from build123d import *

# Parameters (mm, degrees)
SKETCH1_R           = 25
SKETCH1_R_2         = 1.5
BOSS_EXTRUDE1_DEPTH = 7
FILLET1_R           = 0.4
BOSS_EXTRUDE2_DEPTH = 7
MOVE_FACE1_DEPTH    = 7


# Read off the part's stored shape, not the designer's step: Move Face1
with BuildPart() as part:
    # Sketch1 → Boss-Extrude1 (new body)
    with BuildSketch(Plane.XY):
        Circle(SKETCH1_R)
        Circle(SKETCH1_R_2, mode=Mode.SUBTRACT)
    extrude(amount=BOSS_EXTRUDE1_DEPTH)

    # Sketch2 → Cut-Revolve1 (revolve, cut)
    with BuildSketch(Plane(origin=(0, 0, 0), x_dir=(0, 0, -1), z_dir=(1, 0, 0)), mode=Mode.PRIVATE) as cut_revolve1_sk:
        with BuildLine():
            Line((-7, 25), (-6.139887117, 24.237039248))
            ThreePointArc((-6.139887117, 24.237039248), (-3.5, 23.102184954), (-0.860112883, 24.237039248))
            Line((-0.860112883, 24.237039248), (0, 25))
            Line((0, 25), (-7, 25))
        make_face()
    revolve(cut_revolve1_sk.sketch.rotate(Axis((0, 0, 7), (0, 0, -1)), 90), axis=Axis((0, 0, 7), (0, 0, -1)), mode=Mode.SUBTRACT)

    # Fillet1
    fillet1_edges = [part.edges().sort_by_distance(p)[0] for p in [
        (-25, 0, 0),
        (-25, 0, 7),
    ]]
    fillet(fillet1_edges, radius=FILLET1_R)

    # Sketch3 → Boss-Extrude2 (add, through all)
    with BuildSketch(Plane.XY.offset(7)):
        with BuildLine():
            Line((-1.12, 0.997797575), (1.12, 0.997797575))
            ThreePointArc((1.12, 0.997797575), (0, 1.5), (-1.12, 0.997797575))
        make_face()
    extrude(amount=-BOSS_EXTRUDE2_DEPTH)

    # Move Face1 outline → Move Face1 (cut)
    with BuildSketch(Plane.XY):
        with BuildLine():
            ThreePointArc((-1.314115672, 0.997797575), (0, -1.65), (1.314115672, 0.997797575))
            Line((1.314115672, 0.997797575), (1.12, 0.997797575))
            ThreePointArc((1.12, 0.997797575), (0, -1.5), (-1.12, 0.997797575))
            Line((-1.12, 0.997797575), (-1.314115672, 0.997797575))
        make_face()
    extrude(amount=MOVE_FACE1_DEPTH, mode=Mode.SUBTRACT)


solid = part.part
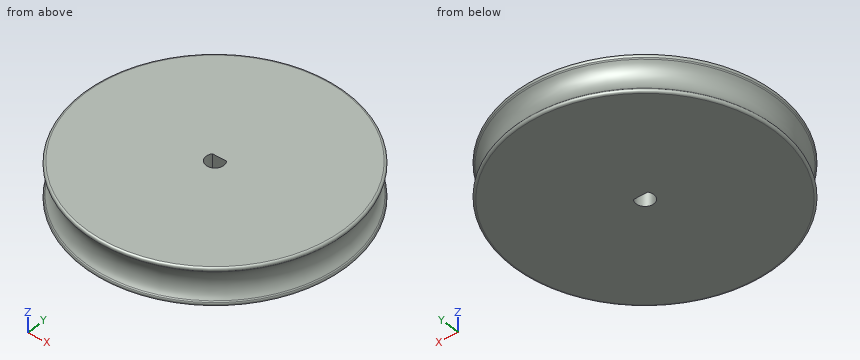
CAD build for the part. Positions are in the model's coordinates, mm. Round coordinates to 2 decimals unless told otherwise and drop trailing zeros. Order: outer loops, then holes, each group sorted by start corner. A loop starts at its lowest first (then second) coordinate and runs counter-clockwise, first axis right, second up. Notation, with made-up numbers: (22, 88.25) -> (41, 88.25) arc R18 cw to (41, 106.25) -> close; hole circle Ø9 at (5.5, -20.75). An arc over 180 degrees is marked (long way). Write each question's results on one line, items separated by ' | '.
1. Cut at A-A (y = 0). Give the cut face in (x, z), plus the area to 3 significant figures.
Findings below:
outline: (-24.41, 0.67) arc R0.4 ccw to (-24.11, 0) -> (-1.65, 0) -> (-1.65, 7) -> (-24.11, 7) arc R0.4 ccw to (-24.41, 6.33) -> (-24.24, 6.14) arc R3.64 cw to (-24.24, 0.86) -> close; (1.65, 0) -> (24.11, 0) arc R0.4 ccw to (24.41, 0.67) -> (24.24, 0.86) arc R3.64 cw to (24.24, 6.14) -> (24.41, 6.33) arc R0.4 ccw to (24.11, 7) -> (1.65, 7) -> close | area: 309 mm²
2. Wall check: line 1 along Z through (x, y) = (22.5, 8.5); line 2 along Y through (x, z) = (0, 2.5); line 3 along Y through (x, z) = (0, 5.5). Give the ranges that are in metal, low to high. Write a range as [from, to].
Findings below:
line 1: z = [0, 1.05], [5.95, 7] | line 2: y = [-23.24, -1.65], [1, 23.24] | line 3: y = [-23.7, -1.65], [1, 23.7]
3. Cut at B-B (x = 0). Give the cut face in (y, z), plus the area to 3 significant figures.
Findings below:
outline: (-24.41, 0.67) arc R0.4 ccw to (-24.11, 0) -> (-1.65, 0) -> (-1.65, 7) -> (-24.11, 7) arc R0.4 ccw to (-24.41, 6.33) -> (-24.24, 6.14) arc R3.64 cw to (-24.24, 0.86) -> close; (1, 0) -> (24.11, 0) arc R0.4 ccw to (24.41, 0.67) -> (24.24, 0.86) arc R3.64 cw to (24.24, 6.14) -> (24.41, 6.33) arc R0.4 ccw to (24.11, 7) -> (1, 7) -> close | area: 313 mm²
4. Flat gauge pins, fed straight in: P1, Ø2, axis at x = 0.5, z = 2, coming from the -Y side; P2, Ø4, axis at y = -14.5, z = 6, coming from the +X side; P3, Ø3, axis at y = 3, z = 3, coming from the +X side. Where does each tip first touch, or does it go through?
Findings below:
P1: stops at y = -24.09 | P2: stops at x = 21.03 | P3: stops at x = 23.53
5. Cut at C-C (z = 3.25). Give the cut face in (x, y), plus the area to 3 significant figures.
Findings below:
outline: circle Ø46.22 at (0, 0); hole (-1.31, 1) arc R1.65 ccw (long way) to (1.31, 1) -> close | area: 1,670 mm²
